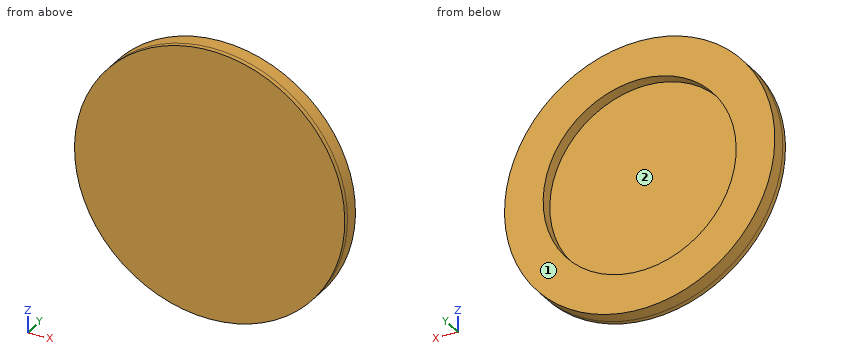
```python
from build123d import *

# Parameters (mm, degrees)
ESBO_O1_R                = 56
ESBO_O1_R_2              = 40
RESSALTO_EXTRUS_O1_DEPTH = 6
RESSALTO_EXTRUS_O2_START = 2
ESBO_O2_R                = 56
RESSALTO_EXTRUS_O2_DEPTH = 2
ESBO_O3_R                = 40
RESSALTO_EXTRUS_O3_DEPTH = 1


with BuildPart() as part:
    # Esboço1 → Ressalto-extrusão1 (new body)
    with BuildSketch(Plane(origin=(0, 0, 0), x_dir=(1, 0, 0), z_dir=(0, 1, 0))):
        with Locations(Location((0, 0, 0), (0, 0, 270))):
            Circle(ESBO_O1_R)
        with Locations(Location((0, 0, 0), (0, 0, 270))):
            Circle(ESBO_O1_R_2, mode=Mode.SUBTRACT)
    extrude(amount=RESSALTO_EXTRUS_O1_DEPTH)

    # Esboço2 → Ressalto-extrusão2 (add)
    with BuildSketch(Plane.XZ.offset(RESSALTO_EXTRUS_O2_START)):
        with Locations(Location((0, 0, 0), (0, 0, 270))):
            Circle(ESBO_O2_R)
    extrude(amount=-RESSALTO_EXTRUS_O2_DEPTH)

    # Esboço3 → Ressalto-extrusão3 (add)
    with BuildSketch(Plane(origin=(0, 0, 0), x_dir=(1, 0, 0), z_dir=(0, 1, 0))):
        with Locations(Location((0, 0, 0), (0, 0, 270))):
            Circle(ESBO_O3_R)
    extrude(amount=RESSALTO_EXTRUS_O3_DEPTH)


solid = part.part
```
Input: part model. Units: mm. Frame: model coordinates. Face numbers are marked on the shaded views. Give positions to 0.01 mm unless a question says otherwise; leave off trailing zeros. Loops run counter-clockwise (first coordinate to the right, second up) from the corner with the lowest first, then second, coordinate; pieces in that order, holes last. Notation, with made-up numbers: (-14, 65) -> (33, 65) arc R21 cw to (33, 89) -> close; hole circle Ø10 at (-3, 52). An arc over 180 degrees is marked (long way). Use a Markdown table: item, result.
Q1. Section query B-B, the plane z = 0. Return the cut outline in (x, y).
Entries:
| item | result |
|---|---|
| outline | (-56, -2) -> (56, -2) -> (56, 6) -> (40, 6) -> (40, 1) -> (-40, 1) -> (-40, 6) -> (-56, 6) -> close |
Q2. Section query D-D, the plane z = -47.5. Return the cut outline in (x, y).
Entries:
| item | result |
|---|---|
| outline | (-29.66, -2) -> (29.66, -2) -> (29.66, 6) -> (-29.66, 6) -> close |
Q3. Ray query, probe 1 along X at (y, z) = (2.7, 0); probe 2 along Y at (x, z) = (24, 4.5); probe 3 along X at (y, z) = (4, 14). Return the intervals inside material, ascending. Write a range as from..to.
Entries:
| item | result |
|---|---|
| probe 1 | x = -56..-40, 40..56 |
| probe 2 | y = -2..1 |
| probe 3 | x = -54.22..-37.47, 37.47..54.22 |
Q4. Section query C-C, the plane y = 3. Return the cut outline in (x, z).
Entries:
| item | result |
|---|---|
| outline | circle Ø112 at (0, 0); hole circle Ø80 at (0, 0) |
Q5. First-contact query: P1, Ø4, axis at y = -0.5, z = -42, coming from the +X side; P2, Ø24, axis at x = -20, z = 0.5, coming from the +Y side; P3, Ø3, axis at y = 3, z = 12, coming from the +X side. Flat tips, straight axial feed; report the tip coordinate or a pass-through.
Entries:
| item | result |
|---|---|
| P1 | stops at x = 39.19 |
| P2 | stops at y = 1 |
| P3 | stops at x = 55.01 |
Q6. Pull-direction query (Z, two-part tool) for the marked faces 1 and 2; classes: pulls with the +Z half, pulls with the -Z half, needs draft (parallel to the pull), parting line crosses it, or undercut.
Entries:
| item | result |
|---|---|
| face 1 | needs draft |
| face 2 | undercut |
Q7. Section query A-A, the plane x = 0. Return the cut outline in (y, z).
Entries:
| item | result |
|---|---|
| outline | (-2, -56) -> (6, -56) -> (6, -40) -> (1, -40) -> (1, 40) -> (6, 40) -> (6, 56) -> (-2, 56) -> close |
